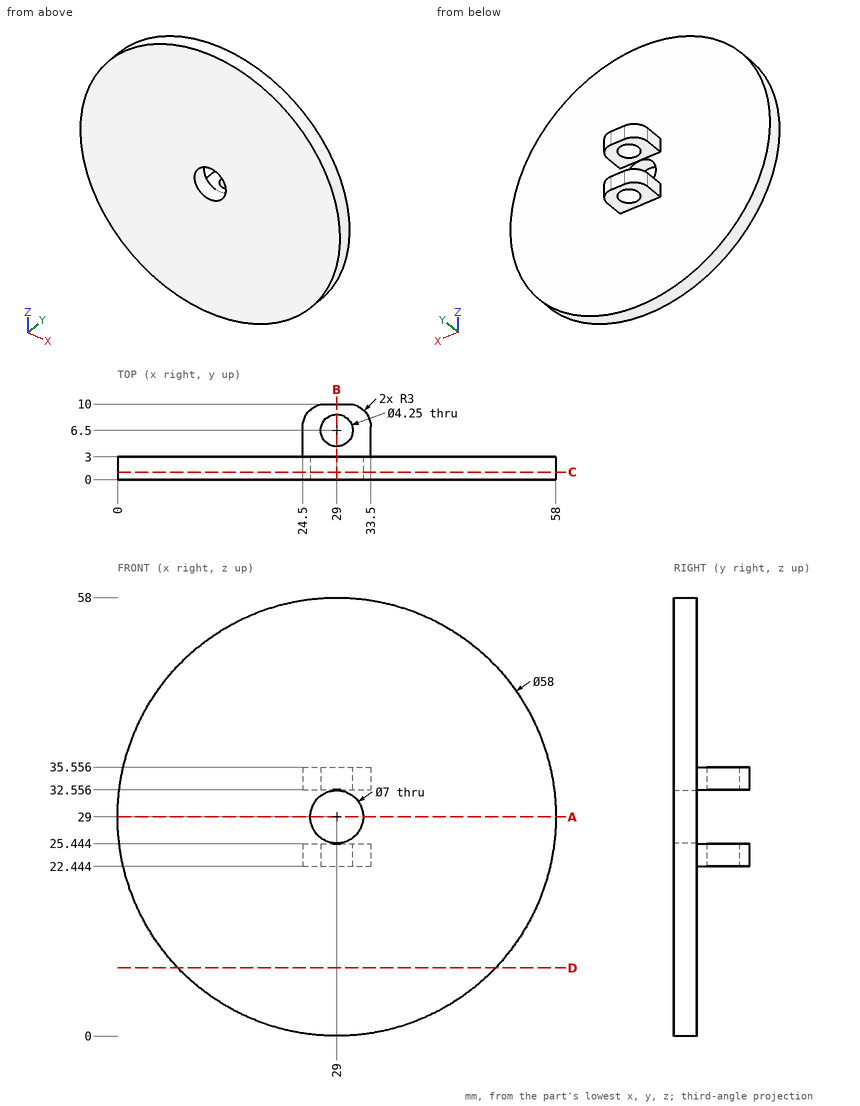
Verification items for this drawing (mm, ordinates from the low corner). Round coordinates to 2 decimals unless told otherwise and drop trailing zeros. Order: outer loops, then holes, each group sorted by start corner. A loop starts at its lowest first (then second) coordinate and runs counter-clockwise, first axis right, second up.
1) Cross-section at A-A, the plane z = 29. Record the cut outline in (x, y), plus the area to 3 significant figures.
Geometry says:
outline: (0, 0) - (25.5, 0) - (25.5, 3) - (0, 3) - close; (32.5, 0) - (58, 0) - (58, 3) - (32.5, 3) - close
area: 153 mm2
2) Cross-section at C-C, the plane y = 1. Record the cut outline in (x, z), plus the area to 3 significant figures.
Geometry says:
outline: circle Ø58 at (29, 29); hole circle Ø7 at (29, 29)
area: 2,600 mm2
3) Depth check by flat-ended pin: pin 1 (5.5 mm diameter, centred on x = 29, y = 6.5, fed in from -Z); pin 2 (3.5 mm diameter, centred on x = 28, y = 5, fed in from +Z); pin 3 (3.5 mm diameter, centred on y = 4, z = 24, fed in from +X). Enter the tip coordinate at first touch or a pass-through.
Geometry says:
pin 1: stops at z = 22.44
pin 2: stops at z = 35.56
pin 3: stops at x = 57.78
4) Cross-section at D-D, the plane z = 9. Record the cut outline in (x, y), plus the area to 3 significant figures.
Geometry says:
outline: (8, 0) - (50, 0) - (50, 3) - (8, 3) - close
area: 126 mm2
5) Cross-section at B-B, the plane x = 29. Give the number of separate pieces and of enclosed holes in the cut face.
Geometry says:
separate pieces: 4
enclosed holes: 0
6) Material ranges on line 1 (X direction, y = 1.95, z = 29); line 2 (Y direction, x = 29, z = 34) (1 decimal); line 3 (Z direction, x = 26.5, y = 6.5) (1 decimal), recorded low to high.
Geometry says:
line 1: x = 0 to 25.5, 32.5 to 58
line 2: y = 0 to 4.4, 8.6 to 10
line 3: z = 22.4 to 25.4, 32.6 to 35.6
